Build history of the part. All positions in model axes, mm. Face numbers are marked on the shaded views. A direction names the side the tool comes from. Coordinates: 2 decimals unless noted, no trailing zeros. Loops run counter-clockwise (first coordinate to the right, second up) from the corner with the lowest first, then second, coordinate; pieces in that order, holes last.
(1) Slice it at D-D (x = -42.5). Give the cut face in (y, z) (3 decimals).
(2) Wall check: L1, parallel to X at y = -23, z = -31 (3 decimals); L2, parallel to Y at x = -42, z = -12.7 (3 decimals); L3, parallel to Y at x = -7, z = -34 (3 decimals). Give the ranges that are in metal, low to high.
(3) Slice it at B-B (x = 10.5). Give the cut face in (y, z) (3 decimals), and give its area (3 significant figures).
(4) Two-plate mould, pull along X, no slides. Class the marked faces 1, 2 and 3: pulls with the +X half, pulls with the -X half, needs draft (parallel to the pull), parting line crosses it, or undercut.
(5) Slice it at A-A (z = -12.7). Give the number of separate pieces and of enclosed holes in the cut face, and give its area (3 significant figures).
(6) Slice it at C-C (z = -31.5). Give the cut face in (x, y) (3 decimals), and give its area (3 significant figures).
(7) Flat gauge pins, fed straight in: P1, Ø6, axis at y = -22.225, z = -12.7, coming from the +X side; P2, Ø1.5, axis at x = -39, y = -15, coming from the -Z side; P3, Ø20, axis at x = -66.5, z = -1, coming from the -Y side (3 decimals); P4, Ø1, axis at y = -29, z = -40, coming from the +X side (3 decimals). Where does each tip first touch, or does it go through?
(8) Tool access for the marked faces 4, 5 and 6: list every direction of +Z, -Z, +X, -X, +Y, -Y with a clear straight run to the whole face (end or side of a thin tool).
from build123d import *

# Parameters (mm, degrees)
SKETCH1_W           = 152.4
SKETCH1_H           = 101.6
BOSS_EXTRUDE1_DEPTH = 9.525
SKETCH2_W           = 9.525
SKETCH2_H           = 101.6
BOSS_EXTRUDE2_DEPTH = 26.67
FILLET1_R           = 1.27
SKETCH3_R           = 3.81
CUT_EXTRUDE1_DEPTH  = 126.095


with BuildPart() as part:
    # Sketch1 → Boss-Extrude1 (new body)
    with BuildSketch(Plane(origin=(0, 0, 0), x_dir=(1, 0, 0), z_dir=(0, 1, 0))):
        Rectangle(SKETCH1_W, SKETCH1_H)
    extrude(amount=-BOSS_EXTRUDE1_DEPTH)

    # Sketch2 → Boss-Extrude2 (add)
    with BuildSketch(Plane.XZ.offset(9.525)):
        with Locations((-44.1325, 0)):
            Rectangle(SKETCH2_W, SKETCH2_H)
        with Locations((44.1325, 0)):
            Rectangle(SKETCH2_W, SKETCH2_H)
    extrude(amount=BOSS_EXTRUDE2_DEPTH)

    # Fillet1
    fillet1_edges = [part.edges().sort_by_distance(p)[0] for p in [
        (-76.2, -9.525, 0),
        (0, -9.525, 50.8),
        (-62.5475, -9.525, -50.8),
        (-39.37, -36.195, 0),
        (-39.37, -22.86, -50.8),
        (-62.5475, -9.525, 50.8),
        (-39.37, -22.86, 50.8),
        (-48.895, -9.525, 0),
        (-48.895, -22.86, 50.8),
        (-48.895, -22.86, -50.8),
        (-44.1325, -36.195, 50.8),
        (-48.895, -36.195, 0),
        (-44.1325, -36.195, -50.8),
        (-39.37, -9.525, 0),
        (62.5475, -9.525, 50.8),
        (0, -9.525, -50.8),
        (48.895, -22.86, 50.8),
        (39.37, -9.525, 0),
        (39.37, -22.86, 50.8),
        (39.37, -22.86, -50.8),
        (48.895, -36.195, 0),
        (48.895, -22.86, -50.8),
        (44.1325, -36.195, 50.8),
        (39.37, -36.195, 0),
        (44.1325, -36.195, -50.8),
        (48.895, -9.525, 0),
        (76.2, -9.525, 0),
        (0, 0, 50.8),
        (-76.2, 0, 0),
        (0, 0, -50.8),
        (76.2, 0, 0),
        (76.2, -4.7625, 50.8),
        (-76.2, -4.7625, 50.8),
        (-76.2, -4.7625, -50.8),
        (76.2, -4.7625, -50.8),
        (62.5475, -9.525, -50.8),
    ]]
    fillet(fillet1_edges, radius=FILLET1_R)

    # Sketch3 → Cut-Extrude1 (cut, through all)
    with BuildSketch(Plane.ZY.offset(48.895)):
        with Locations((12.7, -22.225)):
            Circle(SKETCH3_R)
        with Locations((38.1, -22.225)):
            Circle(SKETCH3_R)
        with Locations((-38.1, -22.225)):
            Circle(SKETCH3_R)
        with Locations((-12.7, -22.225)):
            Circle(SKETCH3_R)
    extrude(amount=-CUT_EXTRUDE1_DEPTH, mode=Mode.SUBTRACT)


solid = part.part
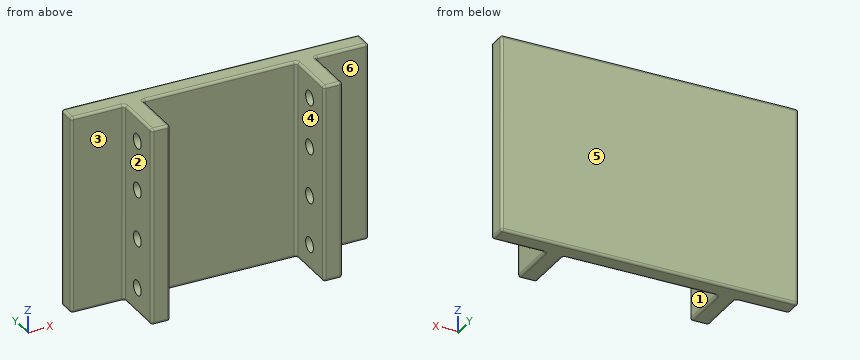
Response values:
1. outline: (-36.195, -49.53) arc R1.27 ccw to (-34.925, -50.8) - (-1.27, -50.8) arc R1.27 ccw to (0, -49.53) - (0, 49.53) arc R1.27 ccw to (-1.27, 50.8) - (-34.925, 50.8) arc R1.27 ccw to (-36.195, 49.53) - close; hole circle Ø7.62 at (-22.225, -38.1); hole circle Ø7.62 at (-22.225, -12.7); hole circle Ø7.62 at (-22.225, 12.7); hole circle Ø7.62 at (-22.225, 38.1)
2. L1: x = -48.895 to -39.37, 39.37 to 48.895
2. L2: y = -36.195 to -26.035, -18.415 to 0
2. L3: y = -9.525 to 0
3. outline: (-9.525, -49.53) arc R1.27 ccw to (-8.255, -50.8) - (-1.27, -50.8) arc R1.27 ccw to (0, -49.53) - (0, 49.53) arc R1.27 ccw to (-1.27, 50.8) - (-8.255, 50.8) arc R1.27 ccw to (-9.525, 49.53) - close
3. area: 966 mm2
4. face 1: undercut
4. face 2: pulls with the -X half
4. face 3: needs draft
5. separate pieces: 3
5. enclosed holes: 0
5. area: 1,810 mm2
6. outline: (-76.2, -8.255) arc R1.27 ccw to (-74.93, -9.525) - (-50.165, -9.525) arc R1.27 cw to (-48.895, -10.795) - (-48.895, -34.925) arc R1.27 ccw to (-47.625, -36.195) - (-40.64, -36.195) arc R1.27 ccw to (-39.37, -34.925) - (-39.37, -10.795) arc R1.27 cw to (-38.1, -9.525) - (38.1, -9.525) arc R1.27 cw to (39.37, -10.795) - (39.37, -34.925) arc R1.27 ccw to (40.64, -36.195) - (47.625, -36.195) arc R1.27 ccw to (48.895, -34.925) - (48.895, -10.795) arc R1.27 cw to (50.165, -9.525) - (74.93, -9.525) arc R1.27 ccw to (76.2, -8.255) - (76.2, -1.27) arc R1.27 ccw to (74.93, 0) - (-74.93, 0) arc R1.27 ccw to (-76.2, -1.27) - close
6. area: 1,960 mm2
7. P1: passes through
7. P2: stops at z = -50.44
7. P3: stops at y = -9.525
7. P4: stops at x = 48.895
8. face 4: +Z, -Z, -Y
8. face 5: +Z, -Z, +X, -X, +Y
8. face 6: +Z, -Z, +X, -Y
